The model under review builds one solid part; all positions refer to its coordinate system, in mm. A direction names the side the tool comes from. Coordinates: 2 decimals unless noted, no trailing zeros. Order: outer loops, then holes, each group sorted by start corner. A loop starts at its lowest first (then second) coordinate and runs counter-clockwise, first axis right, second up. Notation, with made-up numbers: M 81,6.5 L 89,6.5 A21 cw 89,17.5 Z; hole C -32,48.25 d1. An arc over 180 degrees is marked long. One line per item, written item: value.
```python
from build123d import *

# Parameters (mm, degrees)
CUT_EXTRUDE_1_DEPTH      = 16.588457268
CUT_EXTRUDE_1_DEPTH_BACK = 16.588457268
SKETCH_2_W               = 1.6
SKETCH_2_H               = 1
CHAMFER_1_SIZE           = 0.6


with BuildPart() as part:
    # Эскиз1 → Повернуть1 (revolve)
    with BuildSketch(Plane(origin=(0, 0, 0), x_dir=(1, 0, 0), z_dir=(0, 1, 0))):
        Polygon((0, 0), (-3, 0), (-3, 13.700961894), (-0.75, 15), (0, 15), align=None)
    revolve(axis=Axis((0, 0, -15), (0, 0, 1)))

    # Эскиз2 → Вырез-Вытянуть1 (cut, two sides: drawn at the far end of the back side and taken through both)
    with BuildSketch(Plane(origin=(0, 0, 0), x_dir=(0, 0, -1), z_dir=(1, 0, 0)).offset(-CUT_EXTRUDE_1_DEPTH_BACK)):
        with Locations((0.8, 0)):
            Rectangle(SKETCH_2_W, SKETCH_2_H)
    extrude(amount=CUT_EXTRUDE_1_DEPTH + CUT_EXTRUDE_1_DEPTH_BACK, mode=Mode.SUBTRACT)

    # Фаска1
    chamfer_1_edges = [part.edges().sort_by_distance(p)[0] for p in [
        (0, 3, 0),
        (0, -3, 0),
    ]]
    chamfer(chamfer_1_edges, length=CHAMFER_1_SIZE)


solid = part.part
```
(1) We need section C-C, the plane z = -1.75. State the section outline as (x, y) points, plus the area to 3 significant figures.
Geometry results:
outline: C 0,0 d6
area: 28.3 mm2
(2) We need section A-A, the plane y = 0. State the section outline as (x, z) points.
Geometry results:
outline: M -3,-13.7 L -0.75,-15 L 0.75,-15 L 3,-13.7 L 3,-1.6 L -3,-1.6 Z
(3) For L1, parallel to Y at x = 2.05, z = -1.25; L2, parallel to Y at x = -1.25, z = -1.5; L3, parallel to X at y = -0.1, z = -3.75, list the stretches that pass through material, from the lowest coordinate up.
Geometry results:
L1: y = -2.19 to -0.5, 0.5 to 2.19
L2: y = -2.73 to -0.5, 0.5 to 2.73
L3: x = -3 to 3
(4) Tool access review of faces 4 (the flat face through (0, -0.5, -1)), 5 (the flat face through (0, 0, -15)): name each direction out of +Z, -Z, +X, -X, +Y, -Y from which nothing blocks a thin tool from reaching the whole face with its end or side.
Geometry results:
face 4: +Z, +X, -X
face 5: -Z, +X, -X, +Y, -Y
(5) Mouldability with a two-part tool opening along Y and no side actions: class faces 1 (the conical face through (0.1, 2.6, -0.2)), 2 (the flat face through (0, 0.5, -1)), 3 (the cylindrical face through (-2.86, -0.9, -7.24)) as +Y half, -Y half, draft (parallel to the pull), parting line (faces both ways), or undercut.
Geometry results:
face 1: +Y half
face 2: undercut
face 3: parting line
(6) Insertion check: pin 1 Ø3 at (y, z) = (2, -7) entering from -X; pin 2 Ø2 at (x, z) = (1.5, -12.5) entering from +Y; pin 3 Ø0.8 at (x, z) = (-1, -0.5) entering from -Y. Each pin has a flat end and moves straight along its axis. Give the tip position at first contact, or say it passes through.
Geometry results:
pin 1: stops at x = -2.96
pin 2: stops at y = 2.96
pin 3: stops at y = -2.94
(7) We need section B-B, the plane x = 0. State the section outline as (y, z) points, plus the area to 3 significant figures.
Geometry results:
outline: M -3,-13.7 L -0.75,-15 L 0.75,-15 L 3,-13.7 L 3,-0.6 L 2.4,0 L 0.5,0 L 0.5,-1.6 L -0.5,-1.6 L -0.5,0 L -2.4,0 L -3,-0.6 Z
area: 85.1 mm2
